```python
from build123d import *

# Parameters (mm, degrees)
BOSS_EXTRUDE2_DEPTH = 25
SKETCH2_W           = 20
SKETCH2_H           = 5
CUT_EXTRUDE2_DEPTH  = 10
SKETCH3_W           = 20
SKETCH3_H           = 5
CUT_EXTRUDE3_DEPTH  = 10
SKETCH4_R           = 15
BOSS_EXTRUDE3_DEPTH = 15
SKETCH5_R           = 10
CUT_EXTRUDE4_DEPTH  = 10
SKETCH6_R           = 5
CUT_EXTRUDE9_DEPTH  = 300
CUT_EXTRUDE10_DEPTH = 10
SKETCH9_R           = 5
CUT_EXTRUDE11_DEPTH = 70


with BuildPart() as part:
    # Sketch1 → Boss-Extrude2 (new body)
    with BuildSketch(Plane.XY):
        with BuildLine():
            Line((-30, 0), (0, 0))
            ThreePointArc((0, 0), (25, -25), (0, -50))
            Line((0, -50), (-30, -50))
            ThreePointArc((-30, -50), (-55, -25), (-30, 0))
        make_face()
    extrude(amount=BOSS_EXTRUDE2_DEPTH)

    # Sketch2 → Cut-Extrude2 (cut)
    with BuildSketch(Plane.XY.offset(25)):
        with Locations((-15, -2.5)):
            Rectangle(SKETCH2_W, SKETCH2_H)
        with Locations((-15, -47.5)):
            Rectangle(SKETCH2_W, SKETCH2_H)
    extrude(amount=-CUT_EXTRUDE2_DEPTH, mode=Mode.SUBTRACT)

    # Sketch3 → Cut-Extrude3 (cut)
    with BuildSketch(Plane(origin=(0, 0, 0), x_dir=(-1, 0, 0), z_dir=(0, 0, -1))):
        with Locations((15, -2.5)):
            Rectangle(SKETCH3_W, SKETCH3_H)
        with Locations((15, -47.5)):
            Rectangle(SKETCH3_W, SKETCH3_H)
    extrude(amount=-CUT_EXTRUDE3_DEPTH, mode=Mode.SUBTRACT)

    # Sketch4 → Boss-Extrude3 (add)
    with BuildSketch(Plane.XY.offset(25)):
        with Locations((-15, -25)):
            Circle(SKETCH4_R)
    extrude(amount=BOSS_EXTRUDE3_DEPTH)

    # Sketch5 → Cut-Extrude4 (cut)
    with BuildSketch(Plane.XY.offset(40)):
        with Locations((-15, -25)):
            Circle(SKETCH5_R)
    extrude(amount=-CUT_EXTRUDE4_DEPTH, mode=Mode.SUBTRACT)

    # Sketch6 → Cut-Extrude9 (cut)
    with BuildSketch(Plane.XY.offset(30)):
        with Locations((-15, -25)):
            Circle(SKETCH6_R)
    extrude(amount=-CUT_EXTRUDE9_DEPTH, mode=Mode.SUBTRACT)

    # Sketch8 → Cut-Extrude10 (cut)
    with BuildSketch(Plane.XY.offset(25)):
        with BuildLine():
            Line((22.912878475, -35), (12.912878475, -35))
            ThreePointArc((12.912878475, -35), (2.912878475, -25), (12.912878475, -15))
            Line((12.912878475, -15), (22.912878475, -15))
            ThreePointArc((22.912878475, -15), (25, -25), (22.912878475, -35))
        make_face()
        with BuildLine():
            Line((-52.912878475, -15), (-42.912878475, -15))
            ThreePointArc((-42.912878475, -15), (-32.912878475, -25), (-42.912878475, -35))
            Line((-42.912878475, -35), (-52.912878475, -35))
            ThreePointArc((-52.912878475, -35), (-55, -25), (-52.912878475, -15))
        make_face()
    extrude(amount=-CUT_EXTRUDE10_DEPTH, mode=Mode.SUBTRACT)

    # Sketch9 → Cut-Extrude11 (cut)
    with BuildSketch(Plane.XY.offset(15)):
        with Locations((-42.912878475, -25)):
            Circle(SKETCH9_R)
        with Locations((12.912878475, -25)):
            Circle(SKETCH9_R)
    extrude(amount=-CUT_EXTRUDE11_DEPTH, mode=Mode.SUBTRACT)


solid = part.part
```
The model under review builds one solid part; all positions refer to its coordinate system, in mm. A direction names the side the tool comes from. Round coordinates to 2 decimals unless told otherwise and drop trailing zeros. Order: outer loops, then holes, each group sorted by start corner. A loop starts at its lowest first (then second) coordinate and runs counter-clockwise, first axis right, second up.
(1) Take a section at C-C, the plane z = 37. State the section outline as (x, y) points, plus the area to 3 significant figures.
Working result:
outline: circle Ø30 at (-15, -25); hole circle Ø20 at (-15, -25)
area: 393 mm2
(2) Mouldability with a two-part tool opening along Y and no side actions: class faces 6 (the face through (-5, -48, 20)), 7 (the face through (-18.252, -39.643, 32.395)), 8 (the face through (-5.46, -22, 35.07)), 9 (the face through (-15, -5, 5)) as released by +Y, released by -Y, zero draft, split by the parting line, or undercut.
Working result:
face 6: zero draft
face 7: split by the parting line
face 8: undercut
face 9: released by +Y
(3) Wall thickness on L1, parallel to Z at x = -42.5, y = -45; L2, parallel to Y at x = -15, z = 12; L3, parallel to X at y = -46, z = 22: over which ranges is each line inside the solid? List them lowest first.
Working result:
L1: z = 0 to 25
L2: y = -50 to -30, -20 to 0
L3: x = -43.56 to -25, -5 to 13.56
(4) Tool access review of faces 1 (the face through (19, -25, 15)), 2 (the face through (-5, -3, 20)), 3 (the face through (-32.915, -24.78, 20.07)), 4 (the face through (-5, -3, 5)), 5 (the face through (-5, -48, 5)): name each direction out of +Z, -Z, +X, -X, +Y, -Y from which nothing blocks a thin tool from reaching the whole face with its end or side.
Working result:
face 1: +Z, +X
face 2: +Z, +Y
face 3: +Z, -X
face 4: -Z, +Y
face 5: -Z, -Y
(5) For P1, Ø4, axis at y = -48.5, z = 22.5, coming from the -X side; P2, Ø8, axis at y = -45, z = 16, coming from the +X side; P3, Ø4, axis at y = -2.5, z = 20, coming from the +X side; P4, Ø2, axis at x = -32, z = 28, coming from the -Y side, all flat-tipped, find the tip position at first contact; note any pin that passes through.
Working result:
P1: stops at x = -42.76
P2: stops at x = 19.21
P3: stops at x = 14.31
P4: passes through
(6) Take a section at B-B, the plane y = -25. State the section outline as (x, z) points, plus the area to 3 significant figures.
Working result:
outline: (-55, 0) - (-47.91, 0) - (-47.91, 15) - (-55, 15) - close; (-37.91, 0) - (-20, 0) - (-20, 30) - (-25, 30) - (-25, 40) - (-30, 40) - (-30, 25) - (-32.91, 25) - (-32.91, 15) - (-37.91, 15) - close; (-10, 0) - (7.91, 0) - (7.91, 15) - (2.91, 15) - (2.91, 25) - (0, 25) - (0, 40) - (-5, 40) - (-5, 30) - (-10, 30) - close; (17.91, 0) - (25, 0) - (25, 15) - (17.91, 15) - close
area: 1,210 mm2
(7) Take a section at D-D, the plane y = -36. State the section outline as (x, z) points, plus the area to 3 significant figures.
Working result:
outline: (-52.45, 0) - (22.45, 0) - (22.45, 25) - (-4.8, 25) - (-4.8, 40) - (-25.2, 40) - (-25.2, 25) - (-52.45, 25) - close
area: 2,180 mm2
(8) Take a section at A-A, the plane x = -15. State the section outline as (y, z) points, plus the area to 3 significant figures.
Working result:
outline: (-50, 10) - (-45, 10) - (-45, 0) - (-30, 0) - (-30, 30) - (-35, 30) - (-35, 40) - (-40, 40) - (-40, 25) - (-45, 25) - (-45, 15) - (-50, 15) - close; (-20, 0) - (-5, 0) - (-5, 10) - (0, 10) - (0, 15) - (-5, 15) - (-5, 25) - (-10, 25) - (-10, 40) - (-15, 40) - (-15, 30) - (-20, 30) - close
area: 1,000 mm2
